from build123d import *

# Parameters (mm, degrees)
F0_W     = 50.8
F0_H     = 50.8
F1_DEPTH = 50.8
F2_W     = 50.8
F2_H     = 50.8
F2_W_2   = 47.1678
F2_H_2   = 46.9646
F3_DEPTH = 49.53
F4_W     = 46.2026
F4_H     = 46.2026
F5_DEPTH = 48.768


with BuildPart() as f1:
    # F0 (on Front) → F1 (new body)
    with BuildSketch(Plane.XZ):
        with Locations((-25.4, 25.4)):
            Rectangle(F0_W, F0_H)
    extrude(amount=F1_DEPTH)

    # F2 (on face) → F3 (join)
    with BuildSketch(Plane.XZ.offset(50.8)):
        with Locations((-25.4, 25.4)):
            Rectangle(F2_W, F2_H)
        with Locations((-25.302492, 25.391847)):
            Rectangle(F2_W_2, F2_H_2, mode=Mode.SUBTRACT)
    extrude(amount=-F3_DEPTH)

    # F4 (on face) → F5 (cut)
    with BuildSketch(Plane.XZ.offset(50.8)):
        with Locations((-25.401182, 25.392756)):
            Rectangle(F4_W, F4_H)
    extrude(amount=-F5_DEPTH, mode=Mode.SUBTRACT)


solid = f1.part
Build history of the part. All positions in model axes, mm. A direction names the side the tool comes from. Round coordinates to 2 decimals unless told otherwise and drop trailing zeros. Write each loop counter-clockwise with the first axis right and the second up, starting at its lowest first coordinate (ties: lowest second). Pieces come first, ordered by that corner, then holes. Notation, with made-up numbers: M -39,62.5 L 11,62.5 A21 ccw 11,69.5 Z; hole C 85,15.5 d9. An arc over 180 degrees is marked long. Answer in a Markdown table with one row per item.
1. Probe L1, parallel to X at y = -32, z = 22; L2, parallel to Z at x = -21, y = -20; L3, parallel to Y at x = -25, z = 7. List the from-to ranges inside material, lowest first. Write a range as [from, to].
Geometry check:
| item | result |
|---|---|
| L1 | [-50.8, -48.5], [-2.3, 0] |
| L2 | [0, 2.29], [48.49, 50.8] |
| L3 | [-2.03, 0] |
2. Saw through at C-C (x = -36.5). List the corners of the cut face in (y, z).
Geometry check:
| item | result |
|---|---|
| outline | M -50.8,0 L 0,0 L 0,50.8 L -50.8,50.8 L -50.8,48.49 L -2.03,48.49 L -2.03,2.29 L -50.8,2.29 Z |
3. Saw through at A-A (y = -29.5). List the corners of the cut face in (x, z).
Geometry check:
| item | result |
|---|---|
| outline | M -50.8,0 L 0,0 L 0,50.8 L -50.8,50.8 Z; hole M -48.5,2.29 L -2.3,2.29 L -2.3,48.49 L -48.5,48.49 Z |
4. Mould opens along Z. For faces 1 (the face through (-27, -50.8, 1)), 2 (the face through (-26, -27, 48.494)), 3 (the face through (-26, -25, 0)) say: +Z half, -Z half, draft (parallel to the pull), parting line (faces both ways), or undercut.
Geometry check:
| item | result |
|---|---|
| face 1 | draft |
| face 2 | undercut |
| face 3 | -Z half |
5. Flat gauge pin, fed straight in: P1, Ø5, axis at x = -13.5, z = 12.5, coming from the -Y side. Where does the tip first touch, or does it go through?
Geometry check:
| item | result |
|---|---|
| P1 | y = -2.03 |
6. Saw through at B-B (z = 26). List the corners of the cut face in (x, y), and give its area (3 significant figures).
Geometry check:
| item | result |
|---|---|
| outline | M -50.8,-50.8 L -48.5,-50.8 L -48.5,-2.03 L -2.3,-2.03 L -2.3,-50.8 L 0,-50.8 L 0,0 L -50.8,0 Z |
| area | 327 mm2 |
7. Which spindle directions (+Z, -Z, +X, -X, +Y, -Y) get a long thin tool onto all of the face, cutting with end or side? Do faces 4 (the face through (-50.8, -25, 25)), 5 (the face through (-26, -2.032, 26)). Say none if no direction does.
Geometry check:
| item | result |
|---|---|
| face 4 | +Z, -Z, -X, +Y, -Y |
| face 5 | -Y |
